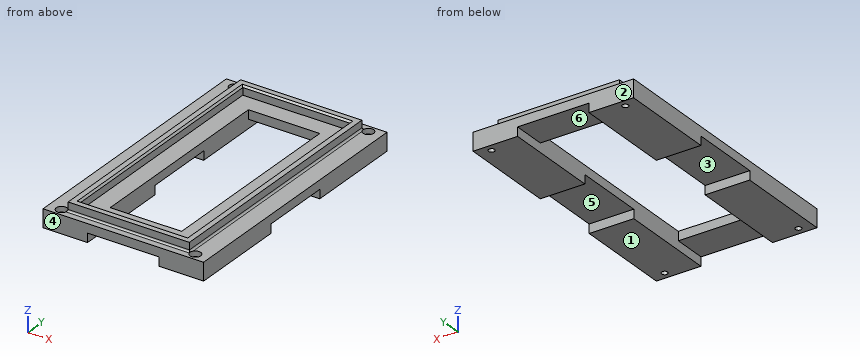
from build123d import *

# Parameters (mm, degrees)
SKETCH1_W           = 90
SKETCH1_H           = 150
BOSS_EXTRUDE1_DEPTH = 10
SKETCH2_W           = 40
SKETCH2_H           = 183.962493804
SKETCH2_W_2         = 287.968551507
SKETCH2_H_2         = 40
CUT_EXTRUDE2_DEPTH  = 5
SKETCH3_R           = 1.7
CUT_EXTRUDE3_DEPTH  = 12
SKETCH4_W           = 68
SKETCH4_H           = 141
SKETCH4_W_2         = 60
SKETCH4_H_2         = 133
BOSS_EXTRUDE2_DEPTH = 5
FILLET1_R           = 1
CHAMFER1_SIZE       = 1
SKETCH5_W           = 40
SKETCH5_H           = 113
CUT_EXTRUDE4_DEPTH  = 10
SKETCH6_R           = 3
SKETCH6_R_2         = 1.7
CUT_EXTRUDE5_DEPTH  = 3


with BuildPart() as part:
    # Sketch1 → Boss-Extrude1 (new body)
    with BuildSketch(Plane.XY):
        with Locations((152.4, 152.4)):
            Rectangle(SKETCH1_W, SKETCH1_H)
    extrude(amount=BOSS_EXTRUDE1_DEPTH)

    # Sketch2 → Cut-Extrude2 (cut)
    with BuildSketch(Plane(origin=(0, 0, 0), x_dir=(-1, 0, 0), z_dir=(0, 0, -1))):
        Polygon((-287.968551507, 162.4), (-287.968551507, 142.4), (-162.4, 142.4), (-162.4, 60.313941127), (-142.4, 60.313941127), (-142.4, 142.4), (0, 142.4), (0, 162.4), (-142.4, 162.4), (-142.4, 244.276434931), (-162.4, 244.276434931), (-162.4, 162.4), align=None)
        with Locations((-152.4, 152.295188029)):
            Rectangle(SKETCH2_W, SKETCH2_H)
        with Locations((-143.984275754, 152.4)):
            Rectangle(SKETCH2_W_2, SKETCH2_H_2)
    extrude(amount=-CUT_EXTRUDE2_DEPTH, mode=Mode.SUBTRACT)

    # Sketch3 → Cut-Extrude3 (cut)
    with BuildSketch(Plane.XY.offset(10)):
        with Locations((189.9, 81.65)):
            Circle(SKETCH3_R)
        with Locations((189.9, 223.15)):
            Circle(SKETCH3_R)
        with Locations((114.9, 223.15)):
            Circle(SKETCH3_R)
        with Locations((114.9, 81.65)):
            Circle(SKETCH3_R)
    extrude(amount=-CUT_EXTRUDE3_DEPTH, mode=Mode.SUBTRACT)

    # Sketch4 → Boss-Extrude2 (add)
    with BuildSketch(Plane.XY.offset(10)):
        with Locations((152.4, 152.4)):
            Rectangle(SKETCH4_W, SKETCH4_H)
        with Locations((152.4, 152.4)):
            Rectangle(SKETCH4_W_2, SKETCH4_H_2, mode=Mode.SUBTRACT)
    extrude(amount=BOSS_EXTRUDE2_DEPTH)

    # Fillet1
    fillet1_edges = [part.edges().sort_by_distance(p)[0] for p in [
        (118.4, 152.4, 10),
        (152.4, 81.9, 10),
        (186.4, 152.4, 10),
        (152.4, 222.9, 10),
    ]]
    fillet(fillet1_edges, radius=FILLET1_R)

    # Chamfer1
    chamfer1_edges = [part.edges().sort_by_distance(p)[0] for p in [
        (152.4, 85.9, 15),
        (182.4, 152.4, 15),
        (152.4, 218.9, 15),
        (122.4, 152.4, 15),
    ]]
    chamfer(chamfer1_edges, length=CHAMFER1_SIZE)

    # Sketch5 → Cut-Extrude4 (cut)
    with BuildSketch(Plane.XY.offset(10)):
        with Locations((152.4, 152.4)):
            Rectangle(SKETCH5_W, SKETCH5_H)
    extrude(amount=-CUT_EXTRUDE4_DEPTH, mode=Mode.SUBTRACT)

    # Sketch6 → Cut-Extrude5 (cut, symmetric)
    # profile 1 of 4: a face of its own
    with BuildSketch(Plane.XY.offset(10)):
        with Locations((114.9, 223.15)):
            Circle(SKETCH6_R)
        with Locations((114.9, 223.15)):
            Circle(SKETCH6_R_2, mode=Mode.SUBTRACT)
    # profile 2 of 4: a face of its own
    with BuildSketch(Plane.XY.offset(10)):
        with Locations((114.9, 81.65)):
            Circle(SKETCH6_R)
        with Locations((114.9, 81.65)):
            Circle(SKETCH6_R_2, mode=Mode.SUBTRACT)
    # profile 3 of 4: a face of its own
    with BuildSketch(Plane.XY.offset(10)):
        with Locations((189.9, 81.65)):
            Circle(SKETCH6_R)
        with Locations((189.9, 81.65)):
            Circle(SKETCH6_R_2, mode=Mode.SUBTRACT)
    # profile 4 of 4: a face of its own
    with BuildSketch(Plane.XY.offset(10)):
        with Locations((189.9, 223.15)):
            Circle(SKETCH6_R)
        with Locations((189.9, 223.15)):
            Circle(SKETCH6_R_2, mode=Mode.SUBTRACT)
    extrude(amount=CUT_EXTRUDE5_DEPTH, both=True, mode=Mode.SUBTRACT)


solid = part.part
For this review, take the finished solid that the model builds, in its own axes (mm). Face numbers are marked on the shaded views. A direction names the side the tool comes from. Round coordinates to 2 decimals unless told otherwise and drop trailing zeros. Write each loop counter-clockwise with the first axis right and the second up, starting at its lowest first coordinate (ties: lowest second). Pieces come first, ordered by that corner, then holes. Notation, with made-up numbers: (57.25, 37.25) -> (86.25, 37.25) arc R34 ccw to (86.25, 68.25) -> close; hole circle Ø5 at (-30, 28). An arc over 180 degrees is marked (long way). Put each result on its own line as item: value.
Q1. Machinability: for the marked faces 4, 5 and 6, which of the approach directions +Z, -Z, +X, -X, +Y, -Y give a long, thin tool a straight path to every point of the face, cutting with its end or side? Answer none if there is none.
Determined:
face 4: +Z, -Z, +X, -X, -Y
face 5: -Z, +X, -X
face 6: -Z, +Y, -Y
Q2. To check wall thickness, follow L1, parallel to X at y = 81.65, z = 3.25; L2, parallel to X at y = 203, z = 2.25; L3, parallel to Y at x = 178.5, z = 3.25. State the ranges of each line that lie inside material, in increasing order. Write a range as [from, to].
Determined:
L1: x = [107.4, 113.2], [116.6, 132.4], [172.4, 188.2], [191.6, 197.4]
L2: x = [107.4, 132.4], [172.4, 197.4]
L3: y = [77.4, 132.4], [172.4, 227.4]
Q3. Consider section D-D on x = 138. State the section outline as (y, z) points, and give its area (3 significant figures).
Determined:
outline: (77.4, 5) -> (95.9, 5) -> (95.9, 10) -> (85.9, 10) -> (85.9, 14) -> (84.9, 15) -> (81.9, 15) -> (81.9, 11) arc R1 cw to (80.9, 10) -> (77.4, 10) -> close; (208.9, 5) -> (227.4, 5) -> (227.4, 10) -> (223.9, 10) arc R1 cw to (222.9, 11) -> (222.9, 15) -> (219.9, 15) -> (218.9, 14) -> (218.9, 10) -> (208.9, 10) -> close
area: 224 mm^2
Q4. Consider section C-C on y = 99.5. State the section outline as (x, z) points, and give its area (3 significant figures).
Determined:
outline: (107.4, 0) -> (132.4, 0) -> (132.4, 10) -> (122.4, 10) -> (122.4, 14) -> (121.4, 15) -> (118.4, 15) -> (118.4, 11) arc R1 cw to (117.4, 10) -> (107.4, 10) -> close; (172.4, 0) -> (197.4, 0) -> (197.4, 10) -> (187.4, 10) arc R1 cw to (186.4, 11) -> (186.4, 15) -> (183.4, 15) -> (182.4, 14) -> (182.4, 10) -> (172.4, 10) -> close
area: 539 mm^2
Q5. The part is to be moulded in two halves that separate along Y. For the marked faces 1, 2 and 3, say which applies: released by +Y, released by -Y, zero draft, split by the parting line, or undercut.
Determined:
face 1: zero draft
face 2: released by +Y
face 3: undercut
Q6. Consider section A-A on z = 2. State the section outline as (x, y) points, and give its area (3 significant figures).
Determined:
outline: (107.4, 77.4) -> (132.4, 77.4) -> (132.4, 132.4) -> (107.4, 132.4) -> close; (107.4, 172.4) -> (132.4, 172.4) -> (132.4, 227.4) -> (107.4, 227.4) -> close; (172.4, 77.4) -> (197.4, 77.4) -> (197.4, 132.4) -> (172.4, 132.4) -> close; (172.4, 172.4) -> (197.4, 172.4) -> (197.4, 227.4) -> (172.4, 227.4) -> close; hole circle Ø3.4 at (114.9, 81.65); hole circle Ø3.4 at (114.9, 223.15); hole circle Ø3.4 at (189.9, 81.65); hole circle Ø3.4 at (189.9, 223.15)
area: 5,460 mm^2
Q7. Clearance check with flat-ended pins moving along their axes: pin 1 Ø3 at (x, y) = (188.5, 83) entering from +Z; pin 2 Ø5 at (x, y) = (113.5, 82.5) entering from +Z; pin 3 Ø1.2 at (x, z) = (155.5, 13) entering from +Y. State where each tip first meets the part, or that it passes through.
Determined:
pin 1: stops at z = 10.08
pin 2: stops at z = 10
pin 3: stops at y = 222.9
Q8. Consider section B-B on x = 114.9. State the section outline as (y, z) points, and give its area (3 significant figures).
Determined:
outline: (77.4, 0) -> (79.95, 0) -> (79.95, 7) -> (78.65, 7) -> (78.65, 10) -> (77.4, 10) -> close; (83.35, 0) -> (132.4, 0) -> (132.4, 5) -> (172.4, 5) -> (172.4, 0) -> (221.45, 0) -> (221.45, 7) -> (220.15, 7) -> (220.15, 10) -> (84.65, 10) -> (84.65, 7) -> (83.35, 7) -> close; (224.85, 0) -> (227.4, 0) -> (227.4, 10) -> (226.15, 10) -> (226.15, 7) -> (224.85, 7) -> close
area: 1,220 mm^2
